The drawing under review shows one solid part. Ordinate dimensions are in mm from its lowest x, y, z. Round coordinates to 2 decimals unless told otherwise and drop trailing zeros. Order: outer loops, then holes, each group sorted by start corner. A loop starts at its lowest first (then second) coordinate and runs counter-clockwise, first axis right, second up. Notation, with made-up numbers: (43.5, 20) - (68.5, 20) arc R15 ccw to (68.5, 44) - close; hole circle Ø11 at (-9, 81.5). An arc over 180 degrees is marked (long way). One line per question, with ' | ' between items.
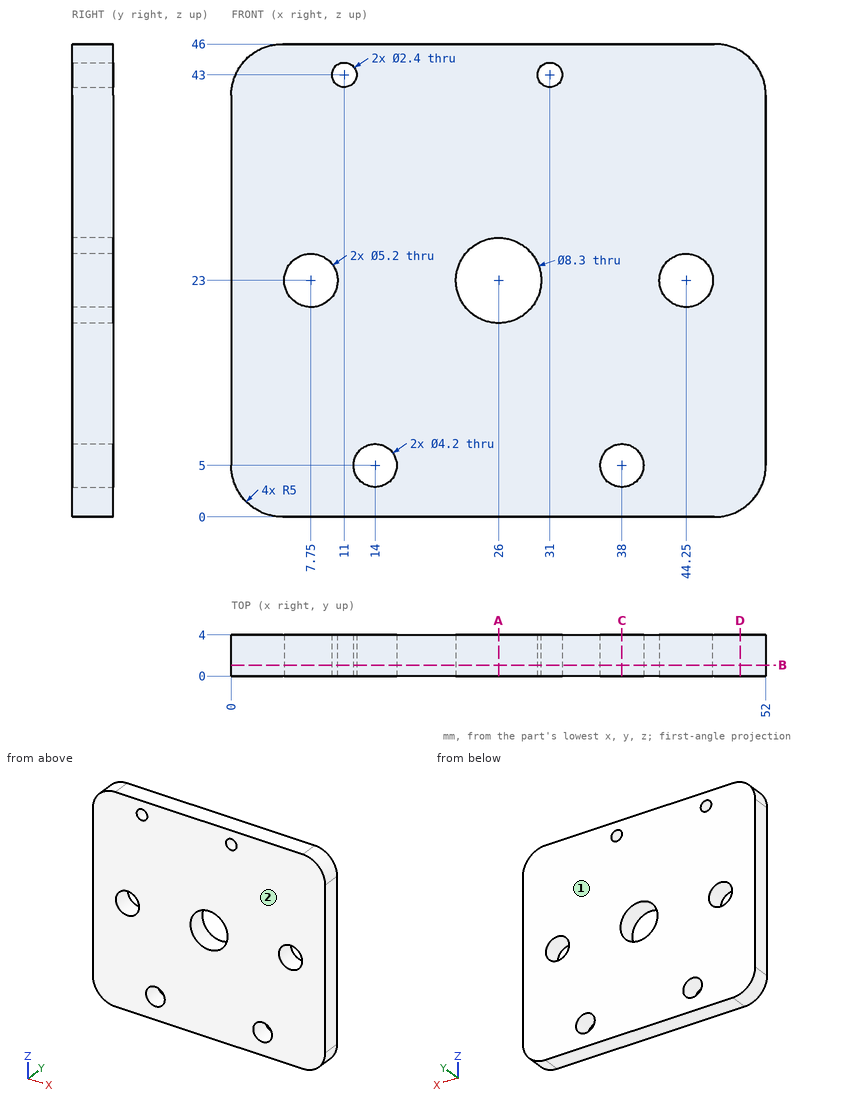
(1) We need section B-B on y = 1.05. State the section outline as (x, z) points.
Output values:
outline: (0, 5) arc R5 ccw to (5, 0) - (47, 0) arc R5 ccw to (52, 5) - (52, 41) arc R5 ccw to (47, 46) - (5, 46) arc R5 ccw to (0, 41) - close; hole circle Ø5.2 at (7.75, 23); hole circle Ø2.4 at (11, 43); hole circle Ø4.2 at (14, 5); hole circle Ø8.3 at (26, 23); hole circle Ø2.4 at (31, 43); hole circle Ø4.2 at (38, 5); hole circle Ø5.2 at (44.25, 23)
(2) Mouldability with a two-part tool opening along Y and no side actions: class the marked faces 1 and 2 as released by +Y, released by -Y, zero draft, split by the parting line, or undercut.
Output values:
face 1: released by +Y | face 2: released by -Y
(3) We need section C-C on x = 38. State the section outline as (y, z) points.
Output values:
outline: (0, 0) - (4, 0) - (4, 2.9) - (0, 2.9) - close; (0, 7.1) - (4, 7.1) - (4, 46) - (0, 46) - close
(4) We need section A-A on x = 26. State the section outline as (y, z) points, plus the area to 3 significant figures.
Output values:
outline: (0, 0) - (4, 0) - (4, 18.85) - (0, 18.85) - close; (0, 27.15) - (4, 27.15) - (4, 46) - (0, 46) - close | area: 151 mm^2
(5) We need section D-D on x = 49.5. State the section outline as (y, z) points.
Output values:
outline: (0, 0.67) - (4, 0.67) - (4, 45.33) - (0, 45.33) - close
(6) For probe 1 along X at (y, z) = (0.4, 5); probe 2 along X at (y, z) = (3, 23); probe 3 along X at (y, z) = (2.4, 43), list the stretches that pass through material, from the lowest coordinate up. Write a range as [from, to].
Output values:
probe 1: [0, 11.9], [16.1, 35.9], [40.1, 52] | probe 2: [0, 5.15], [10.35, 21.85], [30.15, 41.65], [46.85, 52] | probe 3: [0.42, 9.8], [12.2, 29.8], [32.2, 51.58]
